Geometry: final body of the model. Coordinates: model frame, mm. Face numbers are marked on the shaded views. A direction names the side the tool comes from. Give positions to 0.01 mm unless a question says otherwise; leave off trailing zeros. Order: outer loops, then holes, each group sorted by start corner. A loop starts at its lowest first (then second) coordinate and runs counter-clockwise, first axis right, second up. Notation, with made-up numbers: M 61.5,34.5 L 85.5,34.5 A15 ccw 85.5,48.5 Z; hole C 83,37 d6. An arc over 180 degrees is marked long. One line per item, written item: value. Start each with the question number.
```python
from build123d import *

# Parameters (mm, degrees)
F0_W     = 50.8
F0_H     = 50.8
F1_DEPTH = 317.5
F2_W     = 50.8
F2_H     = 38.1
F2_H_2   = 50.8
F3_DEPTH = 12.7
F4_R     = 5.08
F5_D     = 13.49248


with BuildPart() as f1:
    # F0 (on Front) → F1 (new body, symmetric)
    with BuildSketch(Plane.XZ):
        Rectangle(F0_W, F0_H)
    extrude(amount=F1_DEPTH, both=True)

    # F2 (on face) → F3 (join)
    with BuildSketch(Plane.XZ.offset(317.5)):
        with Locations((0, 44.45)):
            Rectangle(F2_W, F2_H)
        Rectangle(F2_W, F2_H_2)
        with Locations((0, -44.45)):
            Rectangle(F2_W, F2_H)
    extrude(amount=F3_DEPTH)

    # F4
    f4_edges = [f1.edges().sort_by_distance(p)[0] for p in [
        (25.4, 0, 25.4),
        (-25.4, 0, 25.4),
        (-25.4, 0, -25.4),
        (25.4, 0, -25.4),
    ]]
    fillet(f4_edges, radius=F4_R)

    # F5 (through all)
    with Locations(Plane(origin=(0, -317.5, 0), x_dir=(1, 0, 0), z_dir=(0, 1, 0))):
        with Locations((0, -50.8), (0, 50.8)):
            Hole(F5_D / 2)

    # F6: F1 across plane


with BuildPart() as f1_1:
    add(f1.part)
    add(f1.part.mirror(Plane.XZ))


solid = f1_1.part
```
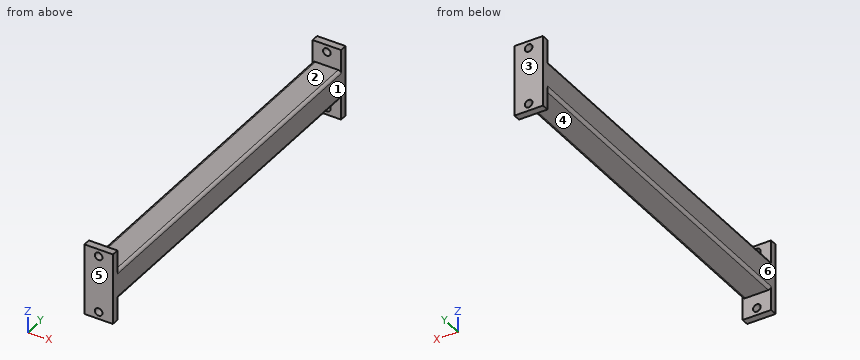
Q1. Contact query for flat-ended pins moving along their axis: pin 1 (11 mm diameter, centred on x = 0, z = 50.8, fed in from -Y); pin 2 (10 mm diameter, centred on x = 15, y = 236, fed in from -Z); pin 3 (2 mm diameter, centred on x = 2, y = 61, fed in from +Z); pin 4 (1 mm diameter, centred on y = 20.5, z = -24, fed in from -X). Output: stop coordinate, or through.
Q2. Section query A-A on x = 0. Return loops of the section in (y, z), and give its area (3 significant figures).
Q3. Section query C-C on y = 269. Return loops of the section in (x, z).
Q4. Mould query, pull axis Y, two halves, no side actions, for the marked faces 3, 4, 5 and 6. Classes: +Y half, -Y half, draft (parallel to the pull), parting line (faces both ways), or undercut.
Q5. Ray query, line 1 along Z through (x, y) = (0, -322); line 2 along Y through (x, z) = (20, 47.5); line 3 along X through (y, z) = (323, -50). Return the intervals inside material, ascending. Write a range as [from, to].
Q6. Section query B-B on z = 50.8. Return loops of the section in (x, y).
Q7. Set-up query: the marked faces 1 and 2. Return all of +Z, -Z, +X, -X, +Y, -Y with unobstructed straight access to the full face (end or side cutting, diameter ignored); none if empty.
Results below:
1. pin 1: through
1. pin 2: z = -25.4
1. pin 3: z = 25.4
1. pin 4: x = -24.28
2. outline: M -330.2,-63.5 L -317.5,-63.5 L -317.5,-57.55 L -330.2,-57.55 Z; M -330.2,-44.05 L -317.5,-44.05 L -317.5,-25.4 L 317.5,-25.4 L 317.5,-44.05 L 330.2,-44.05 L 330.2,44.05 L 317.5,44.05 L 317.5,25.4 L -317.5,25.4 L -317.5,44.05 L -330.2,44.05 Z; M -330.2,57.55 L -317.5,57.55 L -317.5,63.5 L -330.2,63.5 Z; M 317.5,-63.5 L 330.2,-63.5 L 330.2,-57.55 L 317.5,-57.55 Z; M 317.5,57.55 L 330.2,57.55 L 330.2,63.5 L 317.5,63.5 Z
2. area: 34,800 mm2
3. outline: M -25.4,-20.32 A5.08 ccw -20.32,-25.4 L 20.32,-25.4 A5.08 ccw 25.4,-20.32 L 25.4,20.32 A5.08 ccw 20.32,25.4 L -20.32,25.4 A5.08 ccw -25.4,20.32 Z
4. face 3: +Y half
4. face 4: undercut
4. face 5: -Y half
4. face 6: draft
5. line 1: [-63.5, -57.55], [-44.05, 44.05], [57.55, 63.5]
5. line 2: [-330.2, -317.5], [317.5, 330.2]
5. line 3: [-25.4, -6.7], [6.7, 25.4]
6. outline: M -25.4,-330.2 L -6.75,-330.2 L -6.75,-317.5 L -25.4,-317.5 Z; M -25.4,317.5 L -6.75,317.5 L -6.75,330.2 L -25.4,330.2 Z; M 6.75,-330.2 L 25.4,-330.2 L 25.4,-317.5 L 6.75,-317.5 Z; M 6.75,317.5 L 25.4,317.5 L 25.4,330.2 L 6.75,330.2 Z
7. face 1: +Z, -Z, +X, +Y, -Y
7. face 2: +Z, +X, -X
